```python
from build123d import *

# Parameters (mm, degrees)
MAIN_EXTRUSION_DEPTH = 1000


with BuildPart() as part:
    # Sk Main Extrusion → Main Extrusion (new body)
    with BuildSketch(Plane.XY):
        with BuildLine():
            Line((-19.564823375, 0), (-5.70955999, 0))
            ThreePointArc((-5.70955999, 0), (-5.414054203, -1.387221791), (-4.643319426, -2.577883736))
            ThreePointArc((-4.643319426, -2.577883736), (-4.376983545, -3.328515195), (-4.743536233, -4.035637189))
            ThreePointArc((-4.743536233, -4.035637189), (-5.549065057, -5.188573329), (-5.624751834, -6.592998458))
            ThreePointArc((-5.624751834, -6.592998458), (-4.784658148, -8.996464386), (-3.4312327, -11.152999901))
            ThreePointArc((-3.4312327, -11.152999901), (-3.019905527, -11.480142613), (-2.506922203, -11.594425189))
            ThreePointArc((-2.506922203, -11.594425189), (-2.291191076, -8.361169229), (-1.583815224, -5.198875216))
            ThreePointArc((-1.583815224, -5.198875216), (0, -4.027016521), (1.583815224, -5.198875216))
            ThreePointArc((1.583815224, -5.198875216), (2.291191076, -8.361169229), (2.506922203, -11.594425189))
            ThreePointArc((2.506922203, -11.594425189), (3.019905527, -11.480142613), (3.4312327, -11.152999901))
            ThreePointArc((3.4312327, -11.152999901), (4.784658148, -8.996464386), (5.624751834, -6.592998458))
            ThreePointArc((5.624751834, -6.592998458), (5.549065057, -5.188573329), (4.743536233, -4.035637189))
            ThreePointArc((4.743536233, -4.035637189), (4.376983545, -3.328515195), (4.643319426, -2.577883736))
            ThreePointArc((4.643319426, -2.577883736), (5.325853836, -1.584808807), (5.673737659, -0.43110699))
            ThreePointArc((5.673737659, -0.43110699), (5.522041744, 0.119270785), (5.017650904, 0.386697835))
            Line((5.017650904, 0.386697835), (0.673438444, 0.736480319))
            ThreePointArc((0.673438444, 0.736480319), (0.231134607, 1.019470764), (0.218560941, 1.544407122))
            ThreePointArc((0.218560941, 1.544407122), (0.362130691, 2.399619674), (0, 3.187567735))
            ThreePointArc((0, 3.187567735), (-0.338135797, 3.434666121), (-0.747703743, 3.522116267))
            Line((-0.747703743, 3.522116267), (-4.928660874, 3.522116267))
            Line((-4.928660874, 3.522116267), (-17.063386647, 1.866924243))
            ThreePointArc((-17.063386647, 1.866924243), (-18.541135771, 2.274001462), (-19.266905518, 3.624080204))
            Line((-19.266905518, 3.624080204), (-19.642313181, 7.836439756))
            ThreePointArc((-19.642313181, 7.836439756), (-20.182201782, 8.290299862), (-20.638789315, 7.752715895))
            Line((-20.638789315, 7.752715895), (-20.063273376, 0.460660486))
            ThreePointArc((-20.063273376, 0.460660486), (-19.904183245, 0.132801309), (-19.564823375, 0))
        make_face()
    extrude(amount=-MAIN_EXTRUSION_DEPTH)


solid = part.part
```
Source: CAD feature listing. Evaluate the final solid. Frame: model axes, mm. Round coordinates to 2 decimals unless told otherwise and drop trailing zeros. Loops run counter-clockwise (first coordinate to the right, second up) from the corner with the lowest first, then second, coordinate; pieces in that order, holes last.
1. Contact query for flat-ended pins moving along their axis: pin 1 (15 mm diameter, centred on x = -12.5, z = -393, fed in from -Y); pin 2 (5 mm diameter, centred on y = -8, z = -860, fed in from -X); pin 3 (10 mm diameter, centred on x = -16.5, z = -247, fed in from -Y). Output: stop coordinate, or through.
2. Section query A-A on z = -294.5. Output: boundary loops of the cut face in (x, y) (1 decimal), and give its area (3 significant figures).
3. Ray query, L1, parallel to X at y = 7.75, z = -550; L2, parallel to X at y = 5.5, z = -943; L3, parallel to Y at x = -2.75, z = -65.5. Return the intervals inside material, ascending.
4. Section query B-B on x = -12.5. Output: boundary loops of the cut face in (y, z).
Answers below:
1. pin 1: stops at y = -8.52
1. pin 2: stops at x = -5.69
1. pin 3: stops at y = 0
2. outline: (-20.6, 7.8) - (-20.1, 0.5) arc R0.5 ccw to (-19.6, 0) - (-5.7, 0) arc R3.9 ccw to (-4.6, -2.6) arc R1 cw to (-4.7, -4) arc R2.6 ccw to (-5.6, -6.6) arc R11.4 ccw to (-3.4, -11.2) arc R1.2 ccw to (-2.5, -11.6) arc R21.1 cw to (-1.6, -5.2) arc R1.7 cw to (1.6, -5.2) arc R21.1 cw to (2.5, -11.6) arc R1.2 ccw to (3.4, -11.2) arc R11.4 ccw to (5.6, -6.6) arc R2.6 ccw to (4.7, -4) arc R1 cw to (4.6, -2.6) arc R3.9 ccw to (5.7, -0.4) arc R0.7 ccw to (5, 0.4) - (0.7, 0.7) arc R0.6 cw to (0.2, 1.5) arc R1.5 ccw to (0, 3.2) arc R1 ccw to (-0.7, 3.5) - (-4.9, 3.5) - (-17.1, 1.9) arc R1.9 cw to (-19.3, 3.6) - (-19.6, 7.8) arc R0.5 ccw to start
2. area: 150 mm2
3. L1: x = -20.64 to -19.63
3. L2: x = -20.46 to -19.43
3. L3: y = -11.57 to 3.52
4. outline: (0, -1000) - (2.49, -1000) - (2.49, 0) - (0, 0) - close
